Input: part model. Units: mm. Frame: model coordinates. A direction names the side the tool comes from. Give positions to 0.01 mm unless a question says otherwise; leave off trailing zeros. Loops run counter-clockwise (first coordinate to the right, second up) from the corner with the lowest first, then second, coordinate; pieces in that order, holes last.
from build123d import *

# Parameters (mm, degrees)
SKETCH1_W                      = 40
SKETCH1_H                      = 80
BOSS_EXTRUDE1_DEPTH            = 10
SKETCH2_W                      = 10
SKETCH2_H                      = 10
BOSS_EXTRUDE2_DEPTH            = 20
F_1_4_CLEARANCE_HOLE1_D        = 6.5278
F_1_4_CLEARANCE_HOLE1_DEPTH    = 21
F_1_4_CLEARANCE_HOLE1_TIP      = 1.961148974
M3_CLEARANCE_HOLE3_D           = 3.2
M3_CLEARANCE_HOLE4_D           = 3.2
M3_CLEARANCE_HOLE4_ON_FACE_2_D = 3.2


with BuildPart() as part:
    # Sketch1 → Boss-Extrude1 (new body)
    with BuildSketch(Plane(origin=(0, 0, 0), x_dir=(0, 0, -1), z_dir=(1, 0, 0))):
        with Locations((-1086.086956522, 721.739130435)):
            Rectangle(SKETCH1_W, SKETCH1_H)
    extrude(amount=BOSS_EXTRUDE1_DEPTH)

    # Sketch2 → Boss-Extrude2 (add)
    with BuildSketch(Plane(origin=(10, 0, 0), x_dir=(0, 0, -1), z_dir=(1, 0, 0))):
        with Locations((-1086.086956522, 721.739130435)):
            Rectangle(SKETCH2_W, SKETCH2_H)
    extrude(amount=BOSS_EXTRUDE2_DEPTH)

    # 1/4 Clearance Hole1
    with Locations(Plane(origin=(10, 751.739130435, 1086.086956522), x_dir=(0, 0, 1), z_dir=(1, 0, 0))):
        with Locations((0, 0), (0, 60)):
            Hole(F_1_4_CLEARANCE_HOLE1_D / 2, depth=F_1_4_CLEARANCE_HOLE1_DEPTH)
            with Locations((0, 0, -(F_1_4_CLEARANCE_HOLE1_DEPTH + F_1_4_CLEARANCE_HOLE1_TIP / 2))):  # 118° drill point
                Cone(0, F_1_4_CLEARANCE_HOLE1_D / 2, F_1_4_CLEARANCE_HOLE1_TIP, mode=Mode.SUBTRACT)

    # M3 Clearance Hole3 (through all)
    with Locations(Plane(origin=(5, 701.739130435, 1066.086956522), x_dir=(-1, 0, 0), z_dir=(0, 0, -1))):
        with Locations((0, 0), (0, 40)):
            Hole(M3_CLEARANCE_HOLE3_D / 2)

    # M3 Clearance Hole4 (through all)
    with Locations(Plane(origin=(25, 726.739130435, 1085.639739232), x_dir=(0, 0, 1), z_dir=(0, 1, 0))):
        with Locations((0, 0)):
            Hole(M3_CLEARANCE_HOLE4_D / 2)

    # M3 Clearance Hole4 on face 2 (through all)
    with Locations(Plane(origin=(25, 721.739130435, 1081.086956522), x_dir=(-1, 0, 0), z_dir=(0, 0, -1))):
        with Locations((0, 0)):
            Hole(M3_CLEARANCE_HOLE4_ON_FACE_2_D / 2)


solid = part.part
(1) Ray query, probe 1 along Y at (x, z) = (5, 1085.5); probe 2 along Y at (x, z) = (25, 1082.4); probe 3 along Z at (x, y) = (25, 718.3). Return the intervals inside material, ascending.
Values follow:
probe 1: y = 681.74 to 688.53, 694.95 to 700.14, 703.34 to 740.14, 743.34 to 748.53, 754.95 to 761.74
probe 2: y = 716.74 to 720.14, 723.34 to 726.74
probe 3: z = 1081.09 to 1084.04, 1087.24 to 1091.09
(2) Mould query, pull axis Z, two halves, no side actions, for faces 4 (the flat face through (5, 681.739, 1086)), 5 (the flat face through (20, 722, 1081.087)), 6 (the cylindrical face through (4.93, 754.635, 1084.581)), 7 (the flat face through (20, 722, 1091.087)). Classes: +Z half, -Z half, draft (parallel to the pull), parting line (faces both ways), or undercut.
Values follow:
face 4: draft
face 5: -Z half
face 6: undercut
face 7: +Z half
(3) Cut plane C-C (y = 749.5). Return the cut outline in (x, z).
Values follow:
outline: (0, 1066.09) - (10, 1066.09) - (10, 1083.71) - (0, 1083.71) - close; (0, 1088.46) - (10, 1088.46) - (10, 1106.09) - (0, 1106.09) - close
(4) Cut plane B-B (x = 4.25). Return the cut outline in (y, z), and give its area (3 significant figures).
Values follow:
outline: (681.74, 1066.09) - (700.33, 1066.09) - (700.33, 1106.09) - (681.74, 1106.09) - close; (703.15, 1066.09) - (740.33, 1066.09) - (740.33, 1106.09) - (703.15, 1106.09) - close; (743.15, 1066.09) - (761.74, 1066.09) - (761.74, 1106.09) - (743.15, 1106.09) - close; hole circle Ø6.53 at (691.74, 1086.09); hole circle Ø6.53 at (751.74, 1086.09)
area: 2,910 mm2
(5) Cut plane A-A (x = 25). Return the cut outline in (y, z).
Values follow:
outline: (716.74, 1081.09) - (720.14, 1081.09) - (720.14, 1084.04) - (716.74, 1084.04) - close; (716.74, 1087.24) - (720.14, 1087.24) - (720.14, 1091.09) - (716.74, 1091.09) - close; (723.34, 1081.09) - (726.74, 1081.09) - (726.74, 1084.04) - (723.34, 1084.04) - close; (723.34, 1087.24) - (726.74, 1087.24) - (726.74, 1091.09) - (723.34, 1091.09) - close
(6) Pin query (flat end, axial travel): pin 1 Ø2.5 at (x, z) = (25, 1085.64) entering from +Y; pin 2 Ø8 at (x, z) = (19.5, 1086) entering from -Y; pin 3 Ø20 at (y, z) = (703.5, 1076) entering from +X; pin 4 Ø3.5 at (x, y) = (25, 721.74) entering from -Z. Return the tip coordinate at first contact, or that it passes through.
Values follow:
pin 1: passes through
pin 2: stops at y = 716.74
pin 3: stops at x = 10
pin 4: stops at z = 1081.09
(7) Reachability of faces 1 (the flat face through (20, 716.739, 1086)), 2 (the cylindrical face through (5.7, 700.3, 1086.4)), 3 (the flat face through (20, 726.739, 1086)) from +Z, -Z, +X, -X, +Y, -Y: full face, straight path, thin tool, end or side. Return the list, or none.
Values follow:
face 1: +Z, -Z, +X, -Y
face 2: +Z, -Z
face 3: +Z, -Z, +X, +Y
(8) Cut plane D-D (z = 1079). Return the cut outline in (x, y), and give its area (3 significant figures).
Values follow:
outline: (0, 681.74) - (10, 681.74) - (10, 761.74) - (0, 761.74) - close; hole circle Ø3.2 at (5, 701.74); hole circle Ø3.2 at (5, 741.74)
area: 784 mm2
